Design review of the part shown in the three views and the two pictorial views. Dimensions are in mm from the part's minimum x, y and z. Round coordinates to 2 decimals unless told otherwise and drop trailing zeros. Order: outer loops, then holes, each group sorted by start corner. A loop starts at its lowest first (then second) coordinate and runs counter-clockwise, first axis right, second up. Notation, with made-up numbers: (33, 52.25) -> (37, 52.25) arc R22 ccw to (37, 88.25) -> close; hole circle Ø6 at (62, 59). An arc over 180 degrees is marked (long way). Put each result on its own line as item: value. Start each with the question number.
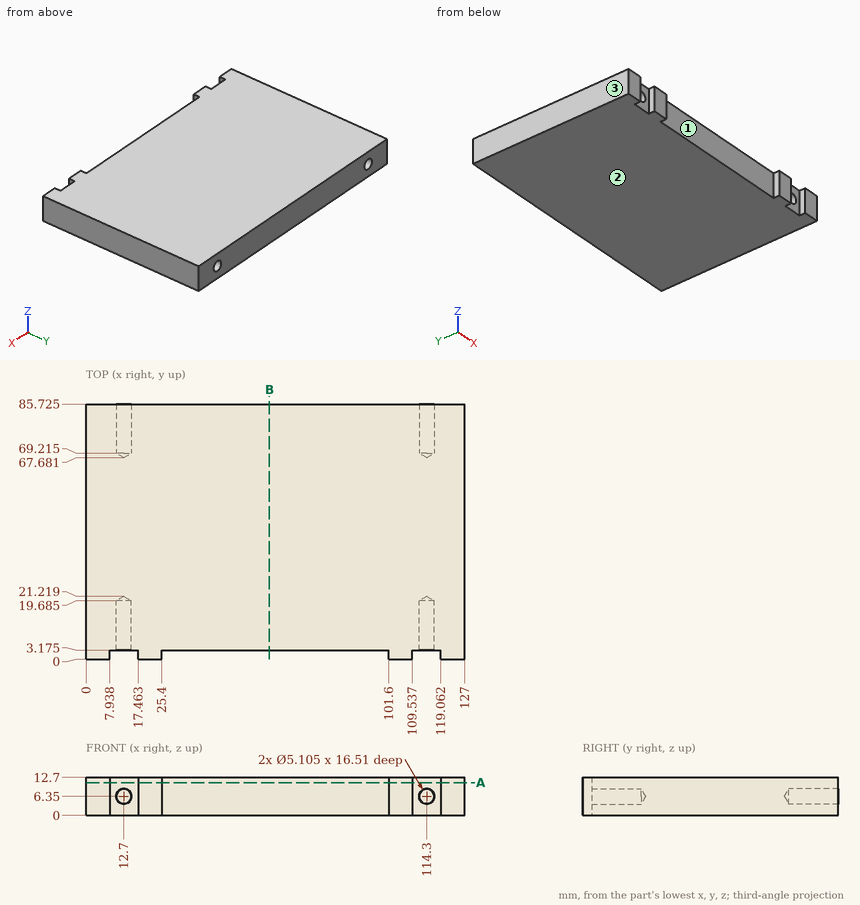
Q1. Take a section at B-B on x = 61.5. Give the boundary of the cut face in (y, z) (1 decimal), and give its area (3 significant figures).
Q2. Take a section at A-A on z = 11. Give the boundary of the cut face in (x, y) (1 decimal).
Q3. Draft analysis for pull direction X (two halves, no side actions). For the marked faces 1, 2 and 3, state which applies: +X half, -X half, draft (parallel to the pull), parting line (faces both ways), or undercut.
Q4. Clearance check with flat-ended pins moving along their axes: pin 1 Ø4 at (x, z) = (114.3, 6.35) entering from -Y; pin 2 Ø1 at (x, z) = (55.5, 8.5) entering from -Y (1 decimal); pin 3 Ø3 at (x, z) = (115, 6.5) entering from -Y. State where each tip first meets the part, or that it passes through.
Q5. Wall thickness on probe 1 along X at (y, z) = (74.5, 6.35); probe 2 along Z at (x, y) = (114.3, 11.5); probe 3 along X at (y, z) = (14, 7.5): over which ranges is each line inside the solid? List them lowest first. Write a range as [from, to].
Calculated:
1. outline: (3.2, 0) -> (85.7, 0) -> (85.7, 12.7) -> (3.2, 12.7) -> close
1. area: 1,050 mm²
2. outline: (0, 0) -> (7.9, 0) -> (7.9, 3.2) -> (17.5, 3.2) -> (17.5, 0) -> (25.4, 0) -> (25.4, 3.2) -> (101.6, 3.2) -> (101.6, 0) -> (109.5, 0) -> (109.5, 3.2) -> (119.1, 3.2) -> (119.1, 0) -> (127, 0) -> (127, 85.7) -> (0, 85.7) -> close
3. face 1: undercut
3. face 2: draft
3. face 3: -X half
4. pin 1: stops at y = 20.02
4. pin 2: stops at y = 3.2
4. pin 3: stops at y = 19.89
5. probe 1: x = [0, 10.15], [15.25, 111.75], [116.85, 127]
5. probe 2: z = [0, 3.8], [8.9, 12.7]
5. probe 3: x = [0, 10.42], [14.98, 112.02], [116.58, 127]
